Study the drawing (mm; zero at the part's minimum x, y, z) and answer. Coordinates: 2 decimals unless noted, no trailing zeros. Write each loop counter-clockwise with the first axis right and the second up, starting at its lowest first coordinate (ties: lowest second). Pieces come first, ordered by that corner, then holes. Notation, with made-up numbers: (-6, 85) -> (34, 85) arc R11 cw to (34, 102) -> close; hole circle Ø8 at (33, -25). An arc over 180 degrees is marked (long way). Answer in a Markdown table with one row per item. Add a question column.
Item 1: Section C-C on y = 65.5 is taken. Write down the section's boundary in (x, z), then the cut area to 3 significant figures.
Item 2: Section D-D on z = 348 is taken. Write down the section's boundary in (x, y).
Item 3: Section B-B on z = 147 is taken. Write down the section's boundary in (x, y).
Item 4: Straight lines are drawn through the part: line 1 (Y direction, x = 40.5, z = 336); line 2 (X direction, y = 71.5, z = 138.5); line 3 (Z direction, x = 5.5, y = 68.5). For each, find the intervals that lie inside material, in ascending order. Write a range as from..to.
Item 5: Given pin 1 Ø5 at (x, z) = (14, 67) entering from +Y; pin 2 Ø13 at (y, z) = (60.5, 185.5) entering from +X; pin 3 Ø13 at (x, y) = (13.5, 70.5) entering from +Z, each flat-ended and moving along its own axis, determine where each tip first touches the part or whether it passes through.
Item 6: Section A-A on x = 6.5 is taken. Write down the section's boundary in (y, z), then the cut area to 3 significant figures.
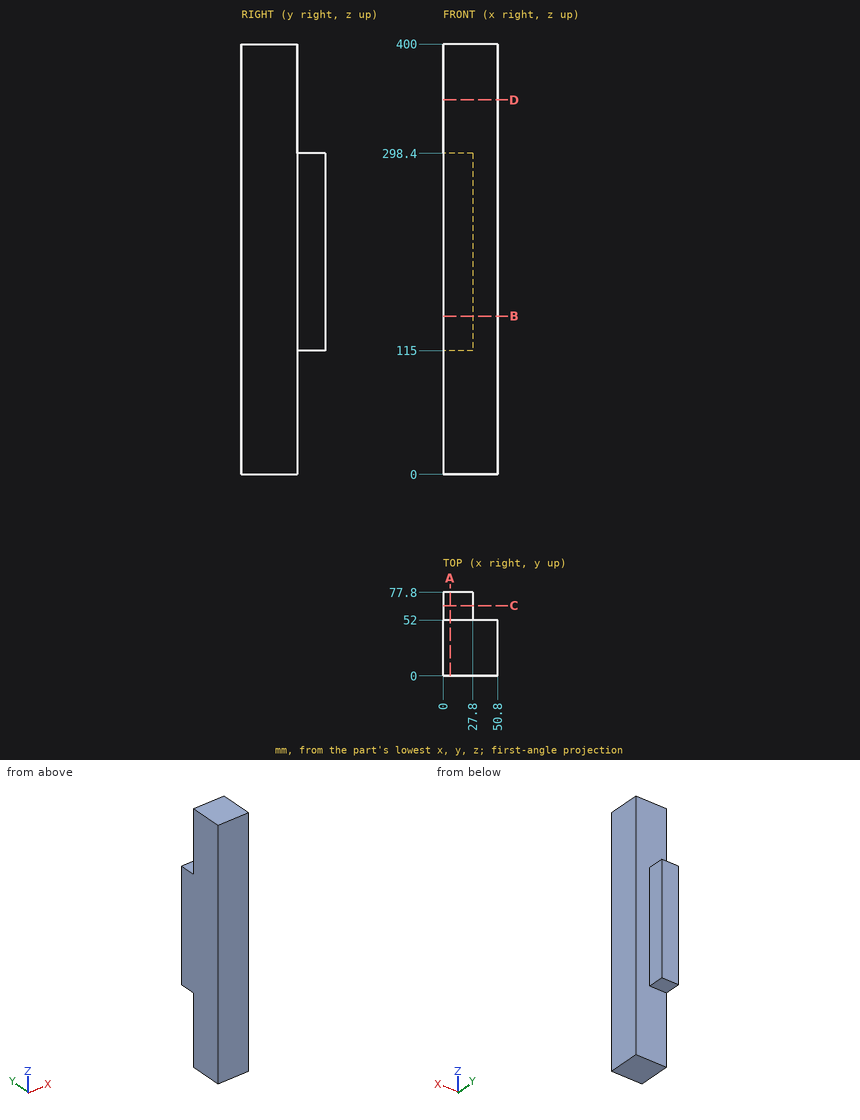
Results below:
| question | item | result |
|---|---|---|
| 1 | outline | (0, 115) -> (27.8, 115) -> (27.8, 298.4) -> (0, 298.4) -> close |
| 1 | area | 5,100 mm2 |
| 2 | outline | (0, 0) -> (50.8, 0) -> (50.8, 52) -> (0, 52) -> close |
| 3 | outline | (0, 0) -> (50.8, 0) -> (50.8, 52) -> (27.8, 52) -> (27.8, 77.8) -> (0, 77.8) -> close |
| 4 | line 1 | y = 0..52 |
| 4 | line 2 | x = 0..27.8 |
| 4 | line 3 | z = 115..298.4 |
| 5 | pin 1 | stops at y = 52 |
| 5 | pin 2 | stops at x = 27.8 |
| 5 | pin 3 | stops at z = 298.4 |
| 6 | outline | (0, 0) -> (52, 0) -> (52, 115) -> (77.8, 115) -> (77.8, 298.4) -> (52, 298.4) -> (52, 400) -> (0, 400) -> close |
| 6 | area | 25,500 mm2 |
